from build123d import *

# Parameters (mm, degrees)
SKETCH1_W           = 1.588
SKETCH1_H           = 1.588
SKETCH1_H_2         = 98.412
SKETCH1_H_3         = 98.4125
SKETCH1_H_4         = 1.5875
BOSS_EXTRUDE1_DEPTH = 25.4


with BuildPart() as part:
    # Sketch1 → Boss-Extrude1 (new body)
    with BuildSketch(Plane(origin=(0, 0, 0), x_dir=(1, 0, 0), z_dir=(0, 1, 0))):
        with BuildLine():
            ThreePointArc((137.441339283, -56), (0, -148.412), (-137.441339283, -56))
            Line((-137.441339283, -56), (-139.154590294, -56))
            ThreePointArc((-139.154590294, -56), (0, -150), (139.154590294, -56))
            Line((139.154590294, -56), (137.441339283, -56))
        make_face()
        with BuildLine():
            Line((103.188, -54.412), (103.188, -56))
            Line((103.188, -56), (137.441339283, -56))
            ThreePointArc((137.441339283, -56), (137.761816422, -55.20691696), (138.077717246, -54.412))
            Line((138.077717246, -54.412), (103.188, -54.412))
        make_face()
        with Locations((102.394, -55.206)):
            Rectangle(SKETCH1_W, SKETCH1_H)
        with Locations((102.394, -5.206)):
            Rectangle(SKETCH1_W, SKETCH1_H_2)
        with Locations((-102.394, -5.20625)):
            Rectangle(SKETCH1_W, SKETCH1_H_3)
        with Locations((-102.394, -55.20625)):
            Rectangle(SKETCH1_W, SKETCH1_H_4)
        with BuildLine():
            Line((-137.441339283, -56), (-103.188, -56))
            Line((-103.188, -56), (-103.188, -54.4125))
            Line((-103.188, -54.4125), (-138.077520211, -54.4125))
            ThreePointArc((-138.077520211, -54.4125), (-137.761716465, -55.207166388), (-137.441339283, -56))
        make_face()
        with BuildLine():
            Line((-139.154590294, -56), (-137.441339283, -56))
            ThreePointArc((-137.441339283, -56), (-137.761716465, -55.207166388), (-138.077520211, -54.4125))
            Line((-138.077520211, -54.4125), (-139.154590294, -54.4125))
            Line((-139.154590294, -54.4125), (-139.154590294, -56))
        make_face()
        with BuildLine():
            ThreePointArc((138.077717246, -54.412), (137.761816422, -55.20691696), (137.441339283, -56))
            Line((137.441339283, -56), (139.154590294, -56))
            Line((139.154590294, -56), (139.154590294, -54.412))
            Line((139.154590294, -54.412), (138.077717246, -54.412))
        make_face()
    extrude(amount=BOSS_EXTRUDE1_DEPTH)


solid = part.part
Could you check a few things on this model? Use its own coordinates, in mm. A direction names the side the tool comes from. Coordinates: 2 decimals unless noted, no trailing zeros. Order: outer loops, then holes, each group sorted by start corner. A loop starts at its lowest first (then second) coordinate and runs counter-clockwise, first axis right, second up.
Q1. Will these pins go through, and if not, where does the flat tip stop? pin 1 (2 mm diameter, centred on x = -90.5, y = 9, fed in from -Z); pin 2 (3 mm diameter, centred on y = 14, z = 37, fed in from +X); pin 3 (1 mm diameter, centred on x = 107, y = 11, fed in from -Z).
Q2. Which directions (+Z, -Z, +X, -X, +Y, -Y) give clear straight access to the entire face, cutting with the end or side of a thin tool? Please do faces 4 (the flat face through (-101.6, 13, 7)), 5 (the flat face through (121, 13, 54.412)), 6 (the flat face through (119, 13, 56)), 7 (the cylindrical face through (-2.5, 12.52, 149.98)).
Q3. Suppose I cut it at C-C on z = 94. Please give me the cut outline in (x, y), and give its area (3 significant figures).
Q4. Suppose I cut it at B-B on y = 8.25. Please give me the cut outline in (x, z).
Q5. Suppose I cut it at A-A on z = 48.5. Please give me the cut outline in (x, y), and give its area (3 significant figures).
Q6. Suppose I cut it at D-D on x = -46. Please give me the cut outline in (y, z).
Q7. Please list where these lines run through material, in increasing order: L1, parallel to X at y = 21, z = 1; L2, parallel to X at y = 6.25, z = 62; L3, parallel to Z at x = 115.5, y = 11.75.
Q8. Thinking about a two-plate mould opening in X: for faces 1 (the flat face through (101.6, 13, 5)), 2 (the flat face through (-121, 13, 54.412)), 3 (the flat face through (-103.188, 13, 5)), which applies, released by +X, released by -X, zero draft, split by the parting line, or undercut?
Answer:
1. pin 1: stops at z = 116.85
1. pin 2: stops at x = 103.19
1. pin 3: stops at z = 54.41
2. face 4: -Z, +Y, -Y
2. face 5: -Z, +X, +Y, -Y
2. face 6: +Y, -Y
2. face 7: +Z, +Y, -Y
3. outline: (-116.89, 0) - (-114.85, 0) - (-114.85, 25.4) - (-116.89, 25.4) - close; (114.85, 0) - (116.89, 0) - (116.89, 25.4) - (114.85, 25.4) - close
3. area: 104 mm2
4. outline: (-139.15, 54.41) - (-103.19, 54.41) - (-103.19, -44) - (-101.6, -44) - (-101.6, 56) - (-137.44, 56) arc R148.41 cw to (137.44, 56) - (101.6, 56) - (101.6, -44) - (103.19, -44) - (103.19, 54.41) - (139.15, 54.41) - (139.15, 56) arc R150 ccw to (-139.15, 56) - close
5. outline: (-103.19, 0) - (-101.6, 0) - (-101.6, 25.4) - (-103.19, 25.4) - close; (101.6, 0) - (103.19, 0) - (103.19, 25.4) - (101.6, 25.4) - close
5. area: 80.7 mm2
6. outline: (0, 141.1) - (25.4, 141.1) - (25.4, 142.77) - (0, 142.77) - close
7. L1: x = -103.19 to -101.6, 101.6 to 103.19
7. L2: x = -136.59 to -134.84, 134.84 to 136.59
7. L3: z = 54.41 to 56, 93.2 to 95.71
8. face 1: undercut
8. face 2: zero draft
8. face 3: released by -X
